Autodesk Inventor part; units mm, degrees
ref_plane "YZ Plane" through (0, 0, 0) normal (1, 0, 0) x (0, 1, 0)
ref_plane "XZ Plane" through (0, 0, 0) normal (0, 1, 0) x (-1, 0, 0)
ref_plane "XY Plane" through (0, 0, 0) normal (0, 0, 1) x (1, 0, 0)
sketch "Эскиз1" plane through (0, 0, 0) normal (0, 0, 1) x (1, 0, 0)
  line L0 (0, 0) -> (0, 20)
  line L1 (0, 20) -> (2.8284, 22.8284)
  line L2 (0, 0) -> (15, 0)
  line L3 (15, 0) -> (15, 20)
  line L4 (15, 20) -> (12.1716, 22.8284)
  line L5 (12.1716, 22.8284) -> (2.8284, 22.8284)
  dimension "d0" = 20
  dimension "d1" = 4
  dimension "d2" = 135
  dimension "d3" = 15
  dimension "d4" = 4
  dimension "d5" = 135
revolve "Вращение1" add sketch "Эскиз1" angle 360 about axis through (0, 0, 0) along (1, 0, 0)
sketch "Эскиз2" plane through (0, 0, 0) normal (-1, 0, 0) x (0, 0, 1)
  point P0 (0, 0)
  point P1 (0, 18)
  point P2 (-15.5885, 9)
  point P3 (-15.5885, -9)
  point P4 (0, -18)
  point P5 (15.5885, -9)
  point P6 (15.5885, 9)
  dimension "d7" = 18
  dimension "d10" = 360
hole "Отверстие1" at (0, 18, 0) at (0, 9, -15.5885) at (0, -9, -15.5885) at (0, -18, 0) at (0, -9, 15.5885) at (0, 9, 15.5885) direction (1, 0, 0) diameter 4 depth 4
sketch "Эскиз3" plane through (15, 0, 0) normal (1, 0, 0) x (0, 0, -1)
  point P0 (0, 0)
  point P1 (0, 14)
  point P2 (-12.1244, 7)
  point P3 (-12.1244, -7)
  point P4 (0, -14)
  point P5 (12.1244, -7)
  point P6 (12.1244, 7)
  dimension "d19" = 14
  dimension "d22" = 360
hole "Отверстие2" at (15, 14, 0) at (15, 7, 12.1244) at (15, -7, 12.1244) at (15, -14, 0) at (15, -7, -12.1244) at (15, 7, -12.1244) direction (-1, 0, 0) diameter 4 depth 4 tip angle 118
sketch "Эскиз4" plane through (0, 0, 0) normal (0, 0, 1) x (1, 0, 0)
  line L0 (0, 0) -> (0, 8)
  line L1 (0, -10) -> (0, 10)
  line L2 (0, 8) -> (0.7, 7.3)
  line L3 (0, 8) -> (0.9899, 8) construction
  line L4 (0.7, 7.3) -> (6.643, 7.3)
  line L5 (6.643, 7.3) -> (6.643, 8)
  line L6 (6.643, 8) -> (7.343, 8)
  line L7 (7.343, 8) -> (7.343, 7.3)
  line L8 (7.343, 7.3) -> (10, 0)
  line L9 (10, 0) -> (0, 0)
  dimension "d31" = 45
  dimension "d32" = 70
  dimension "d33" = 8
  dimension "d35" = 0.7
  dimension "d36" = 0.7
  dimension "d37" = 10
revolve "Вращение2" cut sketch "Эскиз4" angle 360 about axis through (10, 0, 0) along (-1, 0, 0)
properties part number "711136"
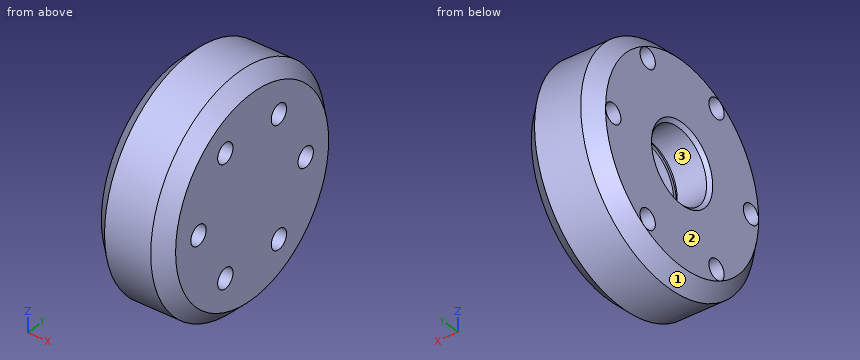
The model under review builds one solid part; all positions refer to its coordinate system, in mm. Face numbers are marked on the shaded views. Round coordinates to 2 decimals unless told otherwise and drop trailing zeros. Write each loop counter-clockwise with the first axis right and the second up, starting at its lowest first coordinate (ties: lowest second). Pieces come first, ordered by that corner, then holes. Notation, with made-up numbers: M -28.5,16 L -6.5,16 A16 ccw -6.5,43 Z; hole C 25.5,14.25 d4. An arc over 180 degrees is marked long. Use a Markdown table: item, result. Add a question column.
Q1. We need section A-A, the plane x = 13.25. State the section outline as (y, z) points, plus the area to 3 significant figures.
Q2. We need section C-C, the plane x = 6. State the section outline as (y, z) points.
Q3. To check wall thickness, follow line 1 (Z direction, x = 2.4, y = 9); line 2 (Z direction, x = 13.9, y = -7); line 3 (Y direction, x = 5.5, z = -2). State the ranges of each line that lie inside material, in increasing order.
Q4. We need section B-B, the plane x = 1.25. State the section outline as (y, z) points, plus the area to 3 significant figures.
Q5. The part is to be moulded in two halves that separate along Y. For the marked faces 1, 2 and 3, say which applies: pulls with the +Y half, pulls with the -Y half, needs draft (parallel to the pull), parting line crosses it, or undercut.
Q6. Insertion check: pin 1 (9 mm diameter, centred on y = 0, z = 0, fed in from -X); pin 2 (1.5 mm diameter, centred on x = 3, y = 18, fed in from -Z); pin 3 (2 mm diameter, centred on x = 2, y = 11, fed in from +Z). Each pin has a flat end and moves straight along its axis. Give the tip position at first contact, or say it passes through.
Findings below:
| question | item | result |
|---|---|---|
| 1 | outline | C 0,0 d43.5; hole C -14,0 d4; hole C -7,-12.12 d4; hole C -7,12.12 d4; hole C 7,-12.12 d4; hole C 7,12.12 d4; hole C 14,0 d4 |
| 1 | area | 1,410 mm² |
| 2 | outline | C 0,0 d45.66; hole C 0,0 d14.6 |
| 3 | line 1 | z = -20.51 to -17.59, -13.59 to 13.59, 17.59 to 20.51 |
| 3 | line 2 | z = -19.91 to -14.12, -10.12 to 10.12, 14.12 to 19.91 |
| 3 | line 3 | y = -22.74 to -7.02, 7.02 to 22.74 |
| 4 | outline | C 0,0 d42.5; hole C -18,0 d4; hole C -9,-15.59 d4; hole C -9,15.59 d4; hole C 0,0 d14.6; hole C 9,-15.59 d4; hole C 9,15.59 d4; hole C 18,0 d4 |
| 4 | area | 1,180 mm² |
| 5 | face 1 | parting line crosses it |
| 5 | face 2 | needs draft |
| 5 | face 3 | undercut |
| 6 | pin 1 | stops at x = 8.36 |
| 6 | pin 2 | stops at z = -14.95 |
| 6 | pin 3 | stops at z = 20.3 |
